CAD build for the part. Positions are in the model's coordinates, mm. A direction names the side the tool comes from. Coordinates: 2 decimals unless noted, no trailing zeros. Write each loop counter-clockwise with the first axis right and the second up, starting at its lowest first coordinate (ties: lowest second). Pieces come first, ordered by that corner, then holes. Notation, with made-up numbers: (30, -20) - (40, -20) arc R5 cw to (40, -14) - close; hole circle Ø10 at (-27, 21.25). An arc over 180 degrees is marked (long way). Answer in a Markdown table with one row per item. Add a question column.
Q1. Pin check, flat tips, straight feed: pin 1 (1 mm diameter, centred on x = 9.5, z = 3.5, fed in from +Y); pin 2 (2 mm diameter, centred on y = -27.5, z = 3, fed in from +X); pin 3 (1.6 mm diameter, centred on x = 7.5, z = 1, fed in from +Y). Stop position of each tip, or through.
Q2. Band-saw the part on D-D (y = -23). List the corners of the cut face in (x, z), and give its area (3 significant figures).
Q3. Band-saw the part on C-C (x = 11.75). List the corners of the cut face in (y, z), and give its area (3 significant figures).
Q4. Drill centre lines: line 1 along Y through (x, z) = (0, 1.4); line 2 along Z through (x, y) = (6.5, 23); line 3 along Y through (x, z) = (-10.75, 1.6). Where is each one in solid material? Low to high. Write a range as from..to.
Q5. Band-saw the part on A-A (x = 0). List the corners of the cut face in (y, z), and give its area (3 significant figures).
Q6. Two-plate mould, pull along X, no slides. Class faces 6 (the flat face through (-6, -27, 3)), 7 (the flat face through (-9, -25.35, 3)), 8 (the cylindrical face through (-0.46, 30.7, 1.01)), 9 (the flat face through (4.75, 30, 1)): +X half, -X half, draft (parallel to the pull), parting line (faces both ways), or undercut.
Q7. 3-axis set-ups, long thin cutter, end or side, ignore diameter. For faces 1 (the flat face through (9, -25.35, 3)), 2 (the flat face through (-10, 27.05, 1)), 3 (the flat face through (-12.5, -27, 3)), 4 (the flat face through (12.5, -27, 3)), 5 (the flat face through (10, 27.05, 1)): which of +Z, -Z, +X, -X, +Y, -Y reach the whole face in a straight line?
Q8. Band-saw the part on B-B (z = 0.9). List the corners of the cut face in (x, y), and give its area (3 significant figures).
```python
from build123d import *

# Parameters (mm, degrees)
SKETCH1_W           = 54.5
SKETCH1_H           = 29.5
BOSS_EXTRUDE1_DEPTH = 2
SKETCH2_W           = 6.5
SKETCH2_H           = 1.9
BOSS_EXTRUDE2_DEPTH = 1.9
SKETCH4_W           = 6.5
SKETCH4_H           = 1.9
BOSS_EXTRUDE3_DEPTH = 1.9
SKETCH5_R           = 2.1
BOSS_EXTRUDE4_DEPTH = 2
SKETCH6_W           = 15.900329316
SKETCH6_H           = 0.2
SKETCH6_W_2         = 14.215882728
CUT_EXTRUDE1_DEPTH  = 10


with BuildPart() as part:
    # Sketch1 → Boss-Extrude1 (new body)
    with BuildSketch(Plane(origin=(0, 0, 0), x_dir=(0, 1, 0), z_dir=(0, 0, 1))):
        Rectangle(SKETCH1_W, SKETCH1_H)
    extrude(amount=BOSS_EXTRUDE1_DEPTH)

    # Sketch2 → Boss-Extrude2 (add, symmetric)
    with BuildSketch(Plane.XZ.offset(27.25)):
        with Locations((-9.25, 2.95)):
            Rectangle(SKETCH2_W, SKETCH2_H)
    extrude(amount=BOSS_EXTRUDE2_DEPTH, both=True)

    # Sketch4 → Boss-Extrude3 (add, symmetric)
    with BuildSketch(Plane.XZ.offset(27.25)):
        with Locations((9.25, 2.95)):
            Rectangle(SKETCH4_W, SKETCH4_H)
    extrude(amount=BOSS_EXTRUDE3_DEPTH, both=True)

    # Sketch5 → Boss-Extrude4 (add)
    with BuildSketch(Plane.XY.offset(2)):
        with BuildLine():
            Line((-4.75, 32.75), (-4.75, 27.25))
            Line((-4.75, 27.25), (4.75, 27.25))
            Line((4.75, 27.25), (4.75, 32.75))
            ThreePointArc((4.75, 32.75), (0, 37.5), (-4.75, 32.75))
        make_face()
        with Locations((0, 32.75)):
            Circle(SKETCH5_R, mode=Mode.SUBTRACT)
    extrude(amount=-BOSS_EXTRUDE4_DEPTH)

    # Sketch6 → Cut-Extrude1 (cut)
    with BuildSketch(Plane.XY.offset(2)):
        with Locations((-12.700164658, 27.15)):
            Rectangle(SKETCH6_W, SKETCH6_H)
        with Locations((11.857941364, 27.15)):
            Rectangle(SKETCH6_W_2, SKETCH6_H)
    extrude(amount=-CUT_EXTRUDE1_DEPTH, mode=Mode.SUBTRACT)


solid = part.part
```
Checked values:
| question | item | result |
|---|---|---|
| 1 | pin 1 | stops at y = -25.35 |
| 1 | pin 2 | stops at x = 12.5 |
| 1 | pin 3 | stops at y = 27.05 |
| 2 | outline | (-14.75, 0) - (14.75, 0) - (14.75, 2) - (-14.75, 2) - close |
| 2 | area | 59.0 mm² |
| 3 | outline | (-29.15, 2) - (-27.25, 2) - (-27.25, 0) - (27.05, 0) - (27.05, 2) - (-25.35, 2) - (-25.35, 3.9) - (-29.15, 3.9) - close |
| 3 | area | 116 mm² |
| 4 | line 1 | y = -27.25..30.65, 34.85..37.5 |
| 4 | line 2 | z = 0..2 |
| 4 | line 3 | y = -27.25..27.05 |
| 5 | outline | (-27.25, 0) - (30.65, 0) - (30.65, 2) - (-27.25, 2) - close; (34.85, 0) - (37.5, 0) - (37.5, 2) - (34.85, 2) - close |
| 5 | area | 121 mm² |
| 6 | face 6 | undercut |
| 6 | face 7 | draft |
| 6 | face 8 | undercut |
| 6 | face 9 | +X half |
| 7 | face 1 | +Z, +X, -X, +Y |
| 7 | face 2 | +Z, -Z, -X, +Y |
| 7 | face 3 | +Z, -X, +Y, -Y |
| 7 | face 4 | +Z, +X, +Y, -Y |
| 7 | face 5 | +Z, -Z, +X, +Y |
| 8 | outline | (-14.75, -27.25) - (14.75, -27.25) - (14.75, 27.05) - (4.75, 27.05) - (4.75, 32.75) arc R4.75 ccw to (-4.75, 32.75) - (-4.75, 27.05) - (-14.75, 27.05) - close; hole circle Ø4.2 at (0, 32.75) |
| 8 | area | 1,680 mm² |
